Build history of the part. All positions in model axes, mm. A direction names the side the tool comes from. Round coordinates to 2 decimals unless told otherwise and drop trailing zeros. Write each loop counter-clockwise with the first axis right and the second up, starting at its lowest first coordinate (ties: lowest second). Pieces come first, ordered by that corner, then holes.
from build123d import *

# Parameters (mm, degrees)
SKETCH1_R                  = 1.5
SHAPE_DEPTH                = 3
MILL_FILLETS_R             = 1
M3_COUNTERSUNKS_AT_2_COUNT = 2
M3_COUNTERSUNKS_AT_2_PITCH = 43.84
M3_COUNTERSUNKS_AT_3_COUNT = 2
M3_COUNTERSUNKS_AT_3_PITCH = 94.086888034
M3_COUNTERSUNKS_AT_4_COUNT = 2
M3_COUNTERSUNKS_AT_4_PITCH = 74.958015582


with BuildPart() as part:
    # Sketch1 → Shape (new body)
    with BuildSketch(Plane(origin=(0, 0, 0), x_dir=(1, 0, 0), z_dir=(0, 1, 0))):
        with BuildLine():
            ThreePointArc((-34.053341195, 38.225), (-36.88, 39.925), (-39.706658805, 38.225))
            Line((-39.706658805, 38.225), (-40.8, 38.225))
            Line((-40.8, 38.225), (-40.8, 35.225))
            Line((-40.8, 35.225), (-39.5, 35.225))
            ThreePointArc((-39.5, 35.225), (-38.5, 34.225), (-39.5, 33.225))
            Line((-39.5, 33.225), (-39.5, -22.225))
            ThreePointArc((-39.5, -22.225), (-38.5, -23.225), (-39.5, -24.225))
            Line((-39.5, -24.225), (-40.8, -24.225))
            Line((-40.8, -24.225), (-40.8, -27.225))
            Line((-40.8, -27.225), (-23.42, -27.225))
            Line((-23.42, -27.225), (-23.42, -33.898341195))
            ThreePointArc((-23.42, -33.898341195), (-21.92, -39.925), (-20.42, -33.898341195))
            Line((-20.42, -33.898341195), (-20.42, -27.225))
            Line((-20.42, -27.225), (-12.393378733, -27.225))
            Line((-12.393378733, -27.225), (0, -11.743815171))
            Line((0, -11.743815171), (12.393378733, -27.225))
            Line((12.393378733, -27.225), (20.42, -27.225))
            Line((20.42, -27.225), (20.42, -33.898341195))
            ThreePointArc((20.42, -33.898341195), (21.92, -39.925), (23.42, -33.898341195))
            Line((23.42, -33.898341195), (23.42, -27.225))
            Line((23.42, -27.225), (40.8, -27.225))
            Line((40.8, -27.225), (40.8, -24.225))
            Line((40.8, -24.225), (39.5, -24.225))
            ThreePointArc((39.5, -24.225), (38.5, -23.225), (39.5, -22.225))
            Line((39.5, -22.225), (39.5, 33.225))
            ThreePointArc((39.5, 33.225), (38.5, 34.225), (39.5, 35.225))
            Line((39.5, 35.225), (40.8, 35.225))
            Line((40.8, 35.225), (40.8, 38.225))
            Line((40.8, 38.225), (39.706658805, 38.225))
            ThreePointArc((39.706658805, 38.225), (36.88, 39.925), (34.053341195, 38.225))
            Line((34.053341195, 38.225), (-34.053341195, 38.225))
        make_face()
        with Locations((36.88, 36.725)):
            Circle(SKETCH1_R, mode=Mode.SUBTRACT)
        Polygon((36.5, -24.225), (13.834640327, -24.225), (1.921447679, -9.343639456), (36.5, 33.850147414), align=None, mode=Mode.SUBTRACT)
        with Locations((-21.92, -36.725)):
            Circle(SKETCH1_R, mode=Mode.SUBTRACT)
        Polygon((-36.5, 33.850147414), (-1.921447679, -9.343639456), (-13.834640327, -24.225), (-36.5, -24.225), align=None, mode=Mode.SUBTRACT)
        with Locations((-36.88, 36.725)):
            Circle(SKETCH1_R, mode=Mode.SUBTRACT)
        Polygon((33.757735438, 35.225), (0, -6.943463741), (-33.757735438, 35.225), align=None, mode=Mode.SUBTRACT)
        with Locations((21.92, -36.725)):
            Circle(SKETCH1_R, mode=Mode.SUBTRACT)
    extrude(amount=SHAPE_DEPTH)

    # Mill fillets
    mill_fillets_edges = [part.edges().sort_by_distance(p)[0] for p in [
        (33.757735438, 1.5, -35.225),
        (-33.757735438, 1.5, -35.225),
        (0, 1.5, 6.943463741),
        (-36.5, 1.5, -33.850147414),
        (-36.5, 1.5, 24.225),
        (-13.834640327, 1.5, 24.225),
        (-1.921447679, 1.5, 9.343639456),
        (36.5, 1.5, -33.850147414),
        (1.921447679, 1.5, 9.343639456),
        (13.834640327, 1.5, 24.225),
        (36.5, 1.5, 24.225),
        (20.42, 1.5, 27.225),
        (12.393378733, 1.5, 27.225),
        (0, 1.5, 11.743815171),
        (-12.393378733, 1.5, 27.225),
        (-20.42, 1.5, 27.225),
        (-23.42, 1.5, 27.225),
        (-39.706658805, 1.5, -38.225),
        (-34.053341195, 1.5, -38.225),
        (34.053341195, 1.5, -38.225),
        (39.706658805, 1.5, -38.225),
        (23.42, 1.5, 27.225),
    ]]
    fillet(mill_fillets_edges, radius=MILL_FILLETS_R)

    # Sketch3 → M3 countersunks (revolve, cut)
    with BuildSketch(Plane(origin=(-21.92, 0, 36.725), x_dir=(0, 0, -1), z_dir=(1, 0, 0))):
        Polygon((0, 0), (0, 3), (1.5, 3), (1.5, 1.7), (3, 0.2), (3, 0), align=None)
    m3_countersunks = revolve(axis=Axis((-21.92, -6.35, 36.725), (0, 1, 0)), mode=Mode.SUBTRACT)

    # M3 countersunks at 2: M3 countersunks ×2
    with Locations(*[(i * M3_COUNTERSUNKS_AT_2_PITCH, 0, 0) for i in range(1, M3_COUNTERSUNKS_AT_2_COUNT)]):
        add(m3_countersunks, mode=Mode.SUBTRACT)

    # M3 countersunks at 3: M3 countersunks ×2
    with Locations(*[Vector(0.624954244, 0, -0.780661382) * (i * M3_COUNTERSUNKS_AT_3_PITCH) for i in range(1, M3_COUNTERSUNKS_AT_3_COUNT)]):
        add(m3_countersunks, mode=Mode.SUBTRACT)

    # M3 countersunks at 4: M3 countersunks ×2
    with Locations(*[Vector(-0.199578389, 0, -0.979881864) * (i * M3_COUNTERSUNKS_AT_4_PITCH) for i in range(1, M3_COUNTERSUNKS_AT_4_COUNT)]):
        add(m3_countersunks, mode=Mode.SUBTRACT)


solid = part.part
1) Slice it at C-C (x = -7.5). Write the cut outline in (y, z) (3 decimals).
Results:
outline: (0, -38.225) - (3, -38.225) - (3, -35.225) - (0, -35.225) - close; (0, -2.425) - (3, -2.425) - (3, 2.375) - (0, 2.375) - close; (0, 16.312) - (3, 16.312) - (3, 21.112) - (0, 21.112) - close
2) Mould opens along X. For faces 1 (the cylindrical face through (35.847, 1.521, -31.939)), 2 (the flat face through (23.42, 1, 31)), 3 (the cylindrical face through (-38.5, 1.5, -34.2)) say: released by +X, released by -X, zero draft, split by the parting line, or undercut.
Results:
face 1: undercut
face 2: released by +X
face 3: released by -X
3) Pin check, flat tips, straight feed: pin 1 Ø0.6 at (x, y) = (-40, 1.5) entering from -Z; pin 2 Ø1 at (x, y) = (-21, 1.5) entering from +Z; pin 3 Ø5 at (x, z) = (-36.88, -36.725) entering from -Y. Stop position of each tip, or through.
Results:
pin 1: stops at z = -38.39
pin 2: stops at z = 39.9
pin 3: stops at y = 0.7
4) Wall check: L1, parallel to X at y = 2.4, z = 24; L2, parallel to X at y = 0.65, z = 11; L3, parallel to Z at x = 3.5, y = 1.4 (3 decimals). Give the ranges that are in metal, low to high.
Results:
L1: x = -38.87 to -36.13, -13.68 to -9.81, 9.81 to 13.68, 36.13 to 38.87
L2: x = -39.5 to -36.5, -3.25 to 3.25, 36.5 to 39.5
L3: z = -38.225 to -35.225, 2.571 to 7.372, 11.315 to 16.116
5) Slice it at A-A (x = 28.5). Write the cut outline in (y, z) (3 decimals), plus the area to 3 significant figures.
Results:
outline: (0, -38.225) - (3, -38.225) - (3, -35.225) - (0, -35.225) - close; (0, -28.657) - (3, -28.657) - (3, -23.857) - (0, -23.857) - close; (0, 24.225) - (3, 24.225) - (3, 27.225) - (0, 27.225) - close
area: 32.4 mm2
6) Which spindle directions (+Z, -Z, +X, -X, +Y, -Y) get a long thin tool onto all of the face, cutting with end or side? Do faces 4 (the flat face through (-18.8, 1.48, -11.74)), 5 (the flat face through (-39.5, 1, -6)), 6 (the flat face through (0, 1, -38.225)). Say none if no direction does.
Results:
face 4: +Y, -Y
face 5: -X, +Y, -Y
face 6: -Z, +Y, -Y
7) Slice it at B-B (z = 17.5). Write the cut outline in (x, y), plus the area to 3 significant figures.
Results:
outline: (-39.5, 0) - (-36.5, 0) - (-36.5, 3) - (-39.5, 3) - close; (-8.45, 0) - (-4.61, 0) - (-4.61, 3) - (-8.45, 3) - close; (4.61, 0) - (8.45, 0) - (8.45, 3) - (4.61, 3) - close; (36.5, 0) - (39.5, 0) - (39.5, 3) - (36.5, 3) - close
area: 41.1 mm2
